from build123d import *

# Parameters (mm, degrees)
F2_SIZE = 0.3175
F3_SIZE = 0.254


with BuildPart() as f1:
    # F0 (on Front) → F1 (revolve)
    with BuildSketch(Plane.XZ):
        Polygon((6.096, 25.4), (6.096, 31.75), (5.30225, 31.75), (0, 25.431025), (0, 0), (6.096, 0), (6.096, 17.4625), (5.7785, 17.4625), (5.7785, 19.05), (6.096, 19.05), (6.096, 20.6375), (5.7785, 20.6375), (5.7785, 22.225), (6.096, 22.225), (6.096, 23.8125), (5.7785, 23.8125), (5.7785, 25.4), align=None)
    revolve(axis=Axis((0, 0, 12.715512), (0, 0, 1)))

    # F2
    f2_edges = [f1.edges().sort_by_distance(p)[0] for p in [
        (-6.096, 0, 31.75),
    ]]
    chamfer(f2_edges, length=F2_SIZE)

    # F3
    f3_edges = [f1.edges().sort_by_distance(p)[0] for p in [
        (-6.096, 0, 25.4),
        (-6.096, 0, 23.8125),
        (-6.096, 0, 22.225),
        (-6.096, 0, 20.6375),
        (-6.096, 0, 19.05),
        (-6.096, 0, 17.4625),
    ]]
    chamfer(f3_edges, length=F3_SIZE)


solid = f1.part
Verification items for the finished model (mm, model axes). A direction names the side the tool comes from. Coordinates: 2 decimals unless noted, no trailing zeros. Loops run counter-clockwise (first coordinate to the right, second up) from the corner with the lowest first, then second, coordinate; pieces in that order, holes last. Notation, with made-up numbers: M 71.25,12.25 L 123.25,12.25 A21 ccw 123.25,22.25 Z; hole C 73.25,66.25 d3. An arc over 180 degrees is marked long. One line per item, written item: value.
1. Section check B-B on z = 16. Record the cut outline in (x, y).
Answers follow:
outline: C 0,0 d12.19
2. Mould release check, pull along X, two halves, no side actions. Record for faces 1 (the cylindrical face through (3.11, 4.87, 24.62)), 2 (the conical face through (1.37, 0.43, 27.14)), 3 (the flat face through (0, 0, 0)): pulls with the +X half, pulls with the -X half, needs draft (parallel to the pull), parting line crosses it, or undercut.
Answers follow:
face 1: parting line crosses it
face 2: undercut
face 3: needs draft
3. Gauge pin test, flat ends, axial feed: P1, Ø3, axis at y = 2, z = 26.5, coming from the -X side; P2, Ø1, axis at y = 3, z = 23, coming from the -X side; P3, Ø3.5, axis at x = -2.5, y = -1, coming from the +Z side. Record the tip position at first contact, or that the pin passes through.
Answers follow:
P1: x = -6.08
P2: x = -5.56
P3: z = 30.73
4. Material ranges on line 1 along Z through (x, y) = (5.5, -2.25); line 2 along Y through (x, z) = (-0.25, 19); line 3 along X through (y, z) = (-0.25, 8), recorded low to high. Write a range as from..to.
Answers follow:
line 1: 0..17.36, 19.15..20.54, 22.33..23.71, 25.5..31.59
line 2: -5.77..5.77
line 3: -6.09..6.09
5. Set-up check for faces 4 (the cylindrical face through (-0.794, 6.044, 28.584)), 5 (the cylindrical face through (3.11, 4.87, 18.27)): record each of +Z, -Z, +X, -X, +Y, -Y from which the full face is reachable in a straight line by a thin tool's end or side.
Answers follow:
face 4: +Z, -Z
face 5: none
6. Section check A-A on z = 24.5. Record the cut outline in (x, y), plus the area to 3 significant figures.
Answers follow:
outline: C 0,0 d11.56
area: 105 mm^2
